Check sheet for the modelled part. Datum: model origin and axes. Units: mm. Coordinates: 2 decimals unless noted, no trailing zeros. Order: outer loops, then holes, each group sorted by start corner. A loop starts at its lowest first (then second) coordinate and runs counter-clockwise, first axis right, second up.
1. Cross-section at B-B (y = 6). Enter the section's corners in (x, z).
2. Thickness scan on line 1 (X direction, y = 6.75, z = -3); line 2 (Z direction, x = -6.5, y = 7.75); line 3 (Y direction, x = -14, z = -27). Record the ranges inside material, lowest first.
3. Gauge pin test, flat ends, axial feed: pin 1 Ø3.5 at (y, z) = (6.5, -5) entering from -X; pin 2 Ø1.2 at (y, z) = (7, -17.5) entering from -X; pin 3 Ø1 at (x, y) = (-3, 1) entering from +Z. Record the tip position at first contact, or that the pin passes through.
4. Cross-section at A-A (z = 0). Count the separate pieces of the cut face and the enclosed holes in it, then the cut area to 3 significant figures.
```python
from build123d import *

# Parameters (mm, degrees)
SKETCH1_RX          = 40
SKETCH1_RY          = 30
BOSS_EXTRUDE1_DEPTH = 5
BOSS_EXTRUDE2_DEPTH = 3
SKETCH3_R           = 1.905
CUT_EXTRUDE1_DEPTH  = 10
SKETCH4_R           = 3.405
CUT_EXTRUDE2_DEPTH  = 3


with BuildPart() as part:
    # Sketch1 → Boss-Extrude1 (new body)
    with BuildSketch(Plane(origin=(0, 0, 0), x_dir=(1, 0, 0), z_dir=(0, 1, 0))):
        with Locations(Location((0, 0), (0, 0, 180))):
            Ellipse(SKETCH1_RX, SKETCH1_RY)
    extrude(amount=BOSS_EXTRUDE1_DEPTH)

    # Sketch2 → Boss-Extrude2 (add)
    with BuildSketch(Plane(origin=(0, 5, 0), x_dir=(1, 0, 0), z_dir=(0, 1, 0))):
        Polygon((-19, 16.5), (-26.5, 16.5), (-26.5, -16.5), (-19, -16.5), (-19, -19), (19, -19), (19, -16.5), (26.5, -16.5), (26.5, 16.5), (19, 16.5), (19, 19), (-19, 19), align=None)
    extrude(amount=BOSS_EXTRUDE2_DEPTH)

    # Sketch3 → Cut-Extrude1 (cut)
    with BuildSketch(Plane.XZ):
        with Locations((32, 0)):
            Circle(SKETCH3_R)
        with Locations((-32, 0)):
            Circle(SKETCH3_R)
    extrude(amount=-CUT_EXTRUDE1_DEPTH, mode=Mode.SUBTRACT)

    # Sketch4 → Cut-Extrude2 (cut)
    with BuildSketch(Plane.XZ):
        with Locations((-32, 0)):
            Circle(SKETCH4_R)
        with Locations((32, 0)):
            Circle(SKETCH4_R)
    extrude(amount=-CUT_EXTRUDE2_DEPTH, mode=Mode.SUBTRACT)


solid = part.part
```
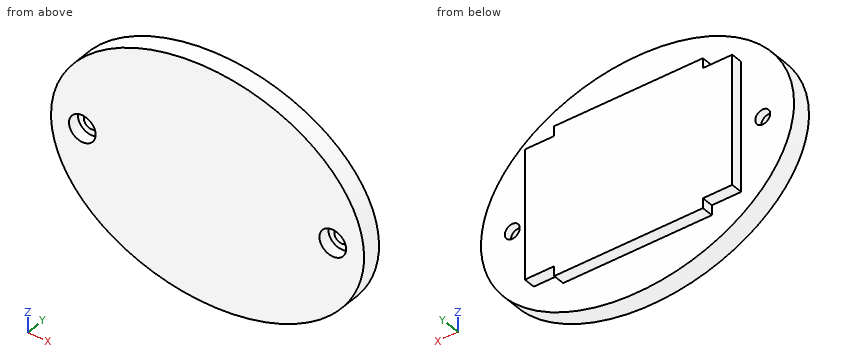
Data:
1. outline: (-26.5, -16.5) - (-19, -16.5) - (-19, -19) - (19, -19) - (19, -16.5) - (26.5, -16.5) - (26.5, 16.5) - (19, 16.5) - (19, 19) - (-19, 19) - (-19, 16.5) - (-26.5, 16.5) - close
2. line 1: x = -26.5 to 26.5
2. line 2: z = -19 to 19
2. line 3: y = 0 to 5
3. pin 1: stops at x = -39.62
3. pin 2: stops at x = -19
3. pin 3: stops at z = 29.94
4. separate pieces: 3
4. enclosed holes: 0
4. area: 503 mm2
